from build123d import *

# Parameters (mm, degrees)
SKETCH1_W           = 29.4
SKETCH1_H           = 5
BOSS_EXTRUDE1_DEPTH = 15.3
CUT_EXTRUDE2_REACH  = 23.799
SKETCH4_W           = 23.4
SKETCH4_H           = 12.3
SKETCH5_W           = 5
SKETCH5_H           = 3
BOSS_EXTRUDE3_DEPTH = 5
CUT_EXTRUDE3_REACH  = 25.359
SKETCH6_R           = 1


with BuildPart() as part:
    # Sketch1 → Boss-Extrude1 (new body)
    with BuildSketch(Plane(origin=(0, 0, 0), x_dir=(1, 0, 0), z_dir=(0, 1, 0))):
        Rectangle(SKETCH1_W, SKETCH1_H)
    extrude(amount=-BOSS_EXTRUDE1_DEPTH)

    # Sketch4 → Cut-Extrude2 (cut, up to next)
    with BuildSketch(Plane.XY.offset(2.5), mode=Mode.PRIVATE) as cut_extrude2_sk1:
        with Locations((0, -9.15)):
            Rectangle(SKETCH4_W, SKETCH4_H)
    cut_extrude2_tool1 = extrude(cut_extrude2_sk1.sketch, amount=-CUT_EXTRUDE2_REACH, mode=Mode.PRIVATE) & part.part
    add(cut_extrude2_tool1.solids().sort_by_distance((0, -9.15, 2.5))[0], mode=Mode.SUBTRACT)

    # Sketch5 → Boss-Extrude3 (add)
    with BuildSketch(Plane(origin=(14.7, 0, 0), x_dir=(0, 0, -1), z_dir=(1, 0, 0))):
        with Locations((0, -13.8)):
            Rectangle(SKETCH5_W, SKETCH5_H)
    boss_extrude3 = extrude(amount=BOSS_EXTRUDE3_DEPTH)

    # Sketch6 → Cut-Extrude3 (cut, up to next)
    with BuildSketch(Plane(origin=(0, -12.3, 0), x_dir=(1, 0, 0), z_dir=(0, 1, 0)), mode=Mode.PRIVATE) as cut_extrude3_sk1:
        with Locations(Location((17.2, 0, 0), (0, 0, 270))):
            Circle(SKETCH6_R)
    cut_extrude3_tool1 = extrude(cut_extrude3_sk1.sketch, amount=-CUT_EXTRUDE3_REACH, mode=Mode.PRIVATE) & part.part
    cut_extrude3 = cut_extrude3_tool1.solids().sort_by_distance((17.2, -12.3, 0))[0]
    add(cut_extrude3, mode=Mode.SUBTRACT)

    # Mirror2: Boss-Extrude3, Cut-Extrude3 across plane
    add(boss_extrude3.mirror(Plane(origin=(0, 0, 0), x_dir=(0, 0, 1), z_dir=(1, 0, 0))))
    add(cut_extrude3.mirror(Plane(origin=(0, 0, 0), x_dir=(0, 0, 1), z_dir=(1, 0, 0))), mode=Mode.SUBTRACT)


solid = part.part
Here's how the part is built. I have some questions about the finished solid (model axes, mm). A direction names the side the tool comes from. Coordinates: 2 decimals unless noted, no trailing zeros. Write each loop counter-clockwise with the first axis right and the second up, starting at its lowest first coordinate (ties: lowest second). Pieces come first, ordered by that corner, then holes.
Item 1: If we mould it in two halves opening along X, with no side actions, what happens to faces 1 (the flat face through (16, -15.3, 0)), 2 (the cylindrical face through (-16.31, -13.78, 0.46)), 3 (the flat face through (-19.7, -14, 0))? For each: +X half, -X half, draft (parallel to the pull), parting line (faces both ways), or undercut.
Item 2: On a 3-axis mill with a long thin cutter (end or side, diameter ignored), from which of +Z, -Z, +X, -X, +Y, -Y can I reach the whole of each face in a straight line? I mean faces 4 (the flat face through (17.16, -12.3, 1.15)), 5 (the flat face through (-14.7, -6, 0)), 6 (the flat face through (11.7, -9, 0)). Say none if no direction works.
Item 3: If I drill on line 1 (X direction, y = -13.7, z = 0); line 2 (X direction, y = -4.25, z = 1.7); line 3 (Z direction, x = -17.2, y = -14.25), over which ranges is the centre line in solid material (lowest first)?
Item 4: I want a section at A-A on y = -9.5. Write out the boundary of the cut face in (x, z), and give its area (3 significant figures).
Item 5: Will these pins go through, and if not, where does the flat tip stop? pin 1 (1 mm diameter, centred on y = -6.5, z = 0, fed in from +X); pin 2 (2 mm diameter, centred on x = 9.5, y = -12, fed in from -Z); pin 3 (2.5 mm diameter, centred on x = -0.5, z = -0.5, fed in from -Y).
Item 6: I want a section at D-D on y = -2. Write out the boundary of the cut face in (x, z), and give its area (3 significant figures).
Item 7: I want a section at C-C on x = -17.2. Write out the boundary of the cut face in (y, z).
Item 8: I want a section at B-B on z = 0. Write out the boundary of the cut face in (x, y), and give its area (3 significant figures).
Findings below:
1. face 1: draft
1. face 2: undercut
1. face 3: -X half
2. face 4: +Z, -Z, +X, +Y
2. face 5: +Z, -Z, -X, +Y
2. face 6: +Z, -Z, -Y
3. line 1: x = -19.7 to -18.2, -16.2 to -11.7, 11.7 to 16.2, 18.2 to 19.7
3. line 2: x = -14.7 to -11.7, 11.7 to 14.7
3. line 3: z = -2.5 to -1, 1 to 2.5
4. outline: (-14.7, -2.5) - (-11.7, -2.5) - (-11.7, 2.5) - (-14.7, 2.5) - close; (11.7, -2.5) - (14.7, -2.5) - (14.7, 2.5) - (11.7, 2.5) - close
4. area: 30.0 mm2
5. pin 1: stops at x = 14.7
5. pin 2: passes through
5. pin 3: stops at y = -3
6. outline: (-14.7, -2.5) - (14.7, -2.5) - (14.7, 2.5) - (-14.7, 2.5) - close
6. area: 147 mm2
7. outline: (-15.3, -2.5) - (-12.3, -2.5) - (-12.3, -1) - (-15.3, -1) - close; (-15.3, 1) - (-12.3, 1) - (-12.3, 2.5) - (-15.3, 2.5) - close
8. outline: (-19.7, -15.3) - (-18.2, -15.3) - (-18.2, -12.3) - (-19.7, -12.3) - close; (-16.2, -15.3) - (-11.7, -15.3) - (-11.7, -3) - (11.7, -3) - (11.7, -15.3) - (16.2, -15.3) - (16.2, -12.3) - (14.7, -12.3) - (14.7, 0) - (-14.7, 0) - (-14.7, -12.3) - (-16.2, -12.3) - close; (18.2, -15.3) - (19.7, -15.3) - (19.7, -12.3) - (18.2, -12.3) - close
8. area: 180 mm2
